```python
from build123d import *

# Parameters (mm, degrees)
F0_W     = 76.2
F0_H     = 88.9
F1_DEPTH = 19.05
F0_H_2   = 25.4
F2_DEPTH = 12.7
F0_W_2   = 127
F0_H_3   = 38.1
F3_DEPTH = 19.05
F4_W     = 79.375
F4_H     = 25.4
F5_DEPTH = 6.35
F6_W     = 76.2
F6_H     = 12.7
F6_W_2   = 79.375
F6_H_2   = 19.05
F7_DEPTH = 6.35
F8_W     = 133.35
F8_H     = 25.4
F8_W_2   = 127
F8_H_2   = 19.05
F9_DEPTH = 6.35


with BuildPart() as f1:
    # F0 (on Front) → F1 (new body)
    with BuildSketch(Plane.XZ):
        with Locations((-177.8, 44.45)):
            Rectangle(F0_W, F0_H)
    extrude(amount=F1_DEPTH)

    # F0 (on Front) → F2 (join)
    with BuildSketch(Plane.XZ):
        with Locations((-101.6, 44.45)):
            Rectangle(F0_W, F0_H)
        with Locations((-101.6, 101.6)):
            Rectangle(F0_W, F0_H_2)
    extrude(amount=F2_DEPTH)



with BuildPart() as f1b:
    # F0 (on Front) → F1, piece 2 (new body)
    with BuildSketch(Plane.XZ):
        with Locations((177.8, 44.45)):
            Rectangle(F0_W, F0_H)
    extrude(amount=F1_DEPTH)

    # F0 (on Front) → F2, piece 2 (join)
    with BuildSketch(Plane.XZ):
        with Locations((101.6, 101.6)):
            Rectangle(F0_W, F0_H_2)
        with Locations((101.6, 44.45)):
            Rectangle(F0_W, F0_H)
    extrude(amount=F2_DEPTH)


with BuildPart() as f1_1:
    add(f1.part)

    add(f1b.part)  # F3 merges F1b
    # F0 (on Front) → F3 (join)
    with BuildSketch(Plane.XZ):
        with Locations((0, 133.35)):
            Rectangle(F0_W_2, F0_H_3)
        with Locations((0, 101.6)):
            Rectangle(F0_W_2, F0_H_2)
        with Locations((0, 44.45)):
            Rectangle(F0_W_2, F0_H)
    extrude(amount=F3_DEPTH)

    # F4 (on face) → F5 (join)
    with BuildSketch(Plane.XY.offset(88.9)):
        Polygon((-139.7, 3.175), (-219.075, 3.175), (-219.075, -22.225), (-139.7, -22.225), (-139.7, -19.05), (-215.9, -19.05), (-215.9, 0), (-139.7, 0), align=None)
        Polygon((-139.7, -12.7), (-139.7, 0), (-215.9, 0), (-215.9, -19.05), (-139.7, -19.05), align=None)
        with Locations((179.3875, -9.525)):
            Rectangle(F4_W, F4_H)
    extrude(amount=F5_DEPTH)

    # F6 (on face) → F7 (join)
    with BuildSketch(Plane.XY.offset(114.3)):
        Polygon((-63.5, 3.175), (-142.875, 3.175), (-142.875, -15.875), (-63.5, -15.875), (-63.5, -12.7), (-139.7, -12.7), (-139.7, 0), (-63.5, 0), align=None)
        with Locations((-101.6, -6.35)):
            Rectangle(F6_W, F6_H)
        with Locations((103.1875, -6.35)):
            Rectangle(F6_W_2, F6_H_2)
    extrude(amount=F7_DEPTH)

    # F8 (on face) → F9 (join)
    with BuildSketch(Plane.XY.offset(152.4)):
        with Locations((0, -9.525)):
            Rectangle(F8_W, F8_H)
        with Locations((0, -9.525)):
            Rectangle(F8_W_2, F8_H_2, mode=Mode.SUBTRACT)
        with Locations((0, -9.525)):
            Rectangle(F8_W_2, F8_H_2)
    extrude(amount=F9_DEPTH)


solid = f1_1.part
```
The listing builds one solid part. Answer for the finished solid, in the listing's coordinates (mm). A direction names the side the tool comes from. Coordinates: 2 decimals unless noted, no trailing zeros. Write each loop counter-clockwise with the first axis right and the second up, starting at its lowest first coordinate (ties: lowest second). Pieces come first, ordered by that corner, then holes. Notation, with made-up numbers: M 54,62.25 L 85,62.25 A7 cw 85,68.25 Z; hole C -1,33.25 d2. An arc over 180 degrees is marked long. Use a Markdown table: item, result. Add a question column.
1. Section A-A (x = 45) is taken. Give the vertices of the cut face in (y, z) (3 decimals), plus the area to 3 significant figures.
2. Section D-D (x = -119) is taken. Give the vertices of the cut face in (y, z) (3 decimals), plus the area to 3 significant figures.
3. Which of the six approach directions +Z, -Z, +X, -X, +Y, -Y give full straight-line access (tool end or side, diameter ignored) to faces 3 (the flat face through (-139.7, -6, 105)), 4 (the flat face through (-215.9, -9, 44)), 5 (the flat face through (215.9, -9, 44)), 6 (the flat face through (63.5, -14, 92)), 7 (the flat face through (139.7, -16, 47))?
4. Straight lines are drawn through the part: line 1 along X through (y, z) = (-17.75, 58.5); line 2 along Z through (x, y) = (-140.5, -5); line 3 along Z through (x, y) = (-71, -2.5). For each, find the intervals that lie inside material, in ascending order. Write a range as [from, to].
5. Section B-B (z = 54) is taken. Give the vertices of the cut face in (x, y), plus the area to 3 significant figures.
6. For a pull along Z with two mould halves and no side action, classify faces 1 (the flat face through (139.7, -6, 105)), 2 (the flat face through (-139.7, -16, 47)) as +Z half, -Z half, draft (parallel to the pull), parting line (faces both ways), or undercut.
7. Section C-C (y = -7) is taken. Give the vertices of the cut face in (x, z) (3 decimals), plus the area to 3 significant figures.
8. Given P1, Ø1, axis at x = 73.5, z = 34, coming from the +Y side; P2, Ø7.5, axis at y = -18.5, z = 43, coming from the +X side; P3, Ø15, axis at y = -6.5, z = 39.5, coming from the -X side, each flat-ended and moving along its own axis, determine where each tip first touches the part or whether it passes through.
Data:
| question | item | result |
|---|---|---|
| 1 | outline | M -22.225,152.4 L -19.05,152.4 L -19.05,0 L 0,0 L 0,152.4 L 3.175,152.4 L 3.175,158.75 L -22.225,158.75 Z |
| 1 | area | 3,060 mm2 |
| 2 | outline | M -15.875,114.3 L -12.7,114.3 L -12.7,0 L 0,0 L 0,114.3 L 3.175,114.3 L 3.175,120.65 L -15.875,120.65 Z |
| 2 | area | 1,570 mm2 |
| 3 | face 3 | -X, +Y, -Y |
| 3 | face 4 | -Z, -X, +Y, -Y |
| 3 | face 5 | -Z, +X, +Y, -Y |
| 3 | face 6 | -Y |
| 3 | face 7 | -Z, -Y |
| 4 | line 1 | x = [-215.9, -139.7], [-63.5, 63.5], [139.7, 215.9] |
| 4 | line 2 | z = [0, 95.25], [114.3, 120.65] |
| 4 | line 3 | z = [0, 120.65] |
| 5 | outline | M -215.9,-19.05 L -139.7,-19.05 L -139.7,-12.7 L -63.5,-12.7 L -63.5,-19.05 L 63.5,-19.05 L 63.5,-12.7 L 139.7,-12.7 L 139.7,-19.05 L 215.9,-19.05 L 215.9,0 L -215.9,0 Z |
| 5 | area | 7,260 mm2 |
| 6 | face 1 | undercut |
| 6 | face 2 | draft |
| 7 | outline | M -219.075,88.9 L -215.9,88.9 L -215.9,0 L 215.9,0 L 215.9,88.9 L 219.075,88.9 L 219.075,95.25 L 139.7,95.25 L 139.7,114.3 L 142.875,114.3 L 142.875,120.65 L 63.5,120.65 L 63.5,152.4 L 66.675,152.4 L 66.675,158.75 L -66.675,158.75 L -66.675,152.4 L -63.5,152.4 L -63.5,120.65 L -142.875,120.65 L -142.875,114.3 L -139.7,114.3 L -139.7,95.25 L -219.075,95.25 Z |
| 7 | area | 53,200 mm2 |
| 8 | P1 | stops at y = 0 |
| 8 | P2 | stops at x = 215.9 |
| 8 | P3 | stops at x = -215.9 |
